```python
from build123d import *

# Parameters (mm, degrees)
SKETCH1_R           = 2
SKETCH1_R_2         = 1.5
SKETCH1_R_3         = 4
BOSS_EXTRUDE1_DEPTH = 2


with BuildPart() as part:
    # Sketch1 → Boss-Extrude1 (new body)
    with BuildSketch(Plane.XY):
        with BuildLine():
            Line((-15, 20), (-15, -20))
            ThreePointArc((-15, -20), (0, -35), (15, -20))
            Line((15, -20), (15, 20))
            ThreePointArc((15, 20), (0, 35), (-15, 20))
        make_face()
        with Locations((0, -25)):
            Circle(SKETCH1_R, mode=Mode.SUBTRACT)
        with Locations((0, -10)):
            Circle(SKETCH1_R, mode=Mode.SUBTRACT)
        with Locations((0, 5)):
            Circle(SKETCH1_R_2, mode=Mode.SUBTRACT)
        with Locations((0, 24)):
            Circle(SKETCH1_R_2, mode=Mode.SUBTRACT)
        with Locations((-8, 14.5)):
            Circle(SKETCH1_R_2, mode=Mode.SUBTRACT)
        with Locations((8, 14.5)):
            Circle(SKETCH1_R_2, mode=Mode.SUBTRACT)
        with Locations((0, 14.5)):
            Circle(SKETCH1_R_3, mode=Mode.SUBTRACT)
        with BuildLine():
            Line((5.656854249, 8.136038969), (8.485281374, 5.307611845))
            ThreePointArc((8.485281374, 5.307611845), (9.192388155, 5.307611845), (9.192388155, 6.014718626))
            Line((9.192388155, 6.014718626), (6.363961031, 8.843145751))
            ThreePointArc((6.363961031, 8.843145751), (5.656854249, 8.843145751), (5.656854249, 8.136038969))
        make_face(mode=Mode.SUBTRACT)
        with BuildLine():
            Line((-6.363961031, 8.843145751), (-9.192388155, 6.014718626))
            ThreePointArc((-9.192388155, 6.014718626), (-9.192388155, 5.307611845), (-8.485281374, 5.307611845))
            Line((-8.485281374, 5.307611845), (-5.656854249, 8.136038969))
            ThreePointArc((-5.656854249, 8.136038969), (-5.656854249, 8.843145751), (-6.363961031, 8.843145751))
        make_face(mode=Mode.SUBTRACT)
        with BuildLine():
            Line((6.363961031, 20.156854249), (9.192388155, 22.985281374))
            ThreePointArc((9.192388155, 22.985281374), (9.192388155, 23.692388155), (8.485281374, 23.692388155))
            Line((8.485281374, 23.692388155), (5.656854249, 20.863961031))
            ThreePointArc((5.656854249, 20.863961031), (5.656854249, 20.156854249), (6.363961031, 20.156854249))
        make_face(mode=Mode.SUBTRACT)
        with BuildLine():
            Line((-5.656854249, 20.863961031), (-8.485281374, 23.692388155))
            ThreePointArc((-8.485281374, 23.692388155), (-9.192388155, 23.692388155), (-9.192388155, 22.985281374))
            Line((-9.192388155, 22.985281374), (-6.363961031, 20.156854249))
            ThreePointArc((-6.363961031, 20.156854249), (-5.656854249, 20.156854249), (-5.656854249, 20.863961031))
        make_face(mode=Mode.SUBTRACT)
    extrude(amount=BOSS_EXTRUDE1_DEPTH)


solid = part.part
```
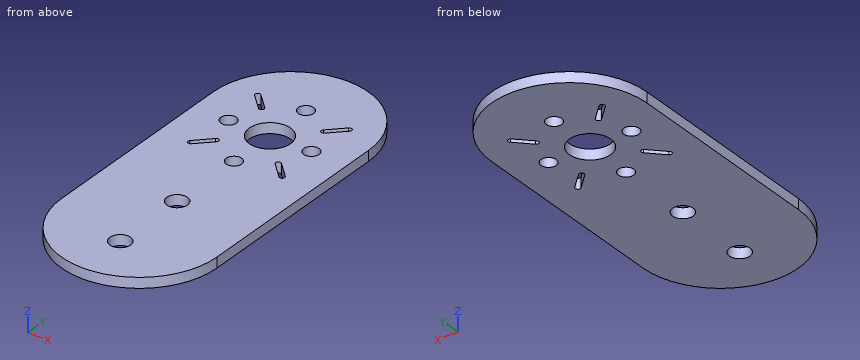
Model file for the job. Use its own axes, mm. Coordinates: 2 decimals unless noted, no trailing zeros. Write each loop counter-clockwise with the first axis right and the second up, starting at its lowest first coordinate (ties: lowest second). Pieces come first, ordered by that corner, then holes. Notation, with made-up numbers: (77.25, 46.5) - (101.25, 46.5) arc R20 ccw to (101.25, 67.5) - close; hole circle Ø9 at (-4.5, 72). An arc over 180 degrees is marked (long way). One line per item, written item: value. Start each with the question number.
1. Slice it at B-B (z = 0.55). Count the separate pieces of the cut face and the enclosed holes in it, plus the area to 3 significant figures.
2. Flat gauge pins, fed straight in: pin 1 (6.5 mm diameter, centred on x = 0, y = 14.5, fed in from +Z); pin 2 (5 mm diameter, centred on x = -8, y = 14.5, fed in from -Z). Where does each tip first touch, or does it go through?
3. Slice it at C-C (x = -7.5). Write the cut outline in (y, z).
4. Slice it at D-D (x = 11). Write the cut outline in (y, z).
5. Probe line 1 (Y direction, x = 0, z = 0.55); line 2 (Y direction, x = -8, z = 1.5); line 3 (Y direction, x = -7.5, z = 0.6). List the from-to ranges inside material, lowest first. Write a range as from..to.
6. Slice it at A-A (x = 0.5). Write the cut outline in (y, z), plus the area to 3 significant figures.
Answers below:
1. separate pieces: 1
1. enclosed holes: 11
1. area: 1,780 mm^2
2. pin 1: passes through
2. pin 2: stops at z = 0
3. outline: (-32.99, 0) - (6.29, 0) - (6.29, 2) - (-32.99, 2) - close; (7.71, 0) - (13.09, 0) - (13.09, 2) - (7.71, 2) - close; (15.91, 0) - (21.29, 0) - (21.29, 2) - (15.91, 2) - close; (22.71, 0) - (32.99, 0) - (32.99, 2) - (22.71, 2) - close
4. outline: (-30.2, 0) - (30.2, 0) - (30.2, 2) - (-30.2, 2) - close
5. line 1: y = -35..-27, -23..-12, -8..3.5, 6.5..10.5, 18.5..22.5, 25.5..35
5. line 2: y = -32.69..5.79, 7.21..13, 16..21.79, 23.21..32.69
5. line 3: y = -32.99..6.29, 7.71..13.09, 15.91..21.29, 22.71..32.99
6. outline: (-34.99, 0) - (-26.94, 0) - (-26.94, 2) - (-34.99, 2) - close; (-23.06, 0) - (-11.94, 0) - (-11.94, 2) - (-23.06, 2) - close; (-8.06, 0) - (3.59, 0) - (3.59, 2) - (-8.06, 2) - close; (6.41, 0) - (10.53, 0) - (10.53, 2) - (6.41, 2) - close; (18.47, 0) - (22.59, 0) - (22.59, 2) - (18.47, 2) - close; (25.41, 0) - (34.99, 0) - (34.99, 2) - (25.41, 2) - close
6. area: 97.3 mm^2
